Autodesk Inventor part; units mm, degrees
ref_plane "YZ Plane" through (0, 0, 0) normal (1, 0, 0) x (0, 1, 0)
ref_plane "XZ Plane" through (0, 0, 0) normal (0, 1, 0) x (-1, 0, 0)
ref_plane "XY Plane" through (0, 0, 0) normal (0, 0, 1) x (1, 0, 0)
sketch "Sketch1" plane through (0, 0, 0) normal (0, 1, 0) x (-1, 0, 0)
  line L0 (-0.2028, 19.4) -> (-0.2028, 32.1) construction
  line L1 (-2.584, 19.4) -> (-2.584, 32.1)
  line L2 (2.1785, 32.1) -> (2.1785, 19.4)
  arc A0 (-2.584, 19.4) -> (2.1785, 19.4) centre (-0.2028, 19.4) ccw
  arc A1 (2.1785, 32.1) -> (-2.584, 32.1) centre (-0.2028, 32.1) ccw
  line L3 (-0.2028, -19.4) -> (-0.2028, -32.1) construction
  line L4 (-2.584, -19.4) -> (-2.584, -32.1)
  line L5 (2.1785, -32.1) -> (2.1785, -19.4)
  arc A2 (2.1785, -19.4) -> (-2.584, -19.4) centre (-0.2028, -19.4) ccw
  arc A3 (-2.584, -32.1) -> (2.1785, -32.1) centre (-0.2028, -32.1) ccw
  line L6 (-51.0028, -76.2) -> (50.5972, -76.2)
  line L7 (50.5972, -76.2) -> (50.5972, 76.2)
  line L8 (50.5972, 76.2) -> (-51.0028, 76.2)
  line L9 (-51.0028, 76.2) -> (-51.0028, -76.2)
  line L10 (-51.0028, -76.2) -> (50.5972, 76.2) construction
  line L11 (50.5972, -76.2) -> (-51.0028, 76.2) construction
  line L12 (50.5972, 76.2) -> (50.5972, 50.8)
  line L13 (50.5972, 50.8) -> (25.1972, 50.8)
  line L14 (-51.0028, 76.2) -> (-51.0028, 50.8)
  line L15 (-51.0028, 50.8) -> (-25.6028, 50.8)
  line L16 (50.5972, -76.2) -> (50.5972, -50.8)
  line L17 (50.5972, -50.8) -> (25.1972, -50.8)
  line L18 (-51.0028, -76.2) -> (-51.0028, -50.8)
  line L19 (-51.0028, -50.8) -> (-25.6028, -50.8)
  circle A4 centre (25.1972, 50.8) radius 2.3813
  circle A5 centre (25.1972, -50.8) radius 2.3812
  circle A6 centre (-25.6028, 50.8) radius 2.3812
  circle A7 centre (-25.6028, -50.8) radius 2.3812
  arc A8 (-2.584, 31.6606) -> (-2.584, -31.6606) centre (-0.2028, 0) ccw
  arc A9 (2.1785, -31.6606) -> (2.1785, 31.6606) centre (-0.2028, 0) ccw
  point P0 (0, 0)
  dimension "d7" = 101.6
  dimension "d8" = 152.4
  dimension "d9" = 25.4
  dimension "d10" = 25.4
  dimension "d11" = 25.4
  dimension "d12" = 25.4
  dimension "d13" = 25.4
  dimension "d14" = 25.4
  dimension "d15" = 25.4
  dimension "d16" = 25.4
  dimension "d17" = 4.7625
  dimension "d18" = 4.7625
  dimension "d19" = 4.7625
  dimension "d20" = 4.7625
extrude "Extrusion1" add sketch "Sketch1" along normal blind 6.35 contours A0 L2 A9 L5 A2 L4 A8 L1 | L9 L8 L7 L6
sketch "Sketch2" plane through (0, 6.35, 0) normal (0, 1, 0) x (1, 0, 0)
  circle A0 centre (0, 0) radius 9.75
  dimension "d23" = 19.5
extrude "Extrusion2" cut sketch "Sketch2" against normal blind 6.35
sketch "Sketch3" plane through (0, 6.35, 0) normal (0, 1, 0) x (1, 0, 0)
  line L0 (-6.6401, -37.7246) -> (10.2278, -37.7246)
  line L1 (10.2278, -37.7246) -> (10.2278, -15.7747)
  line L2 (10.2278, -15.7747) -> (-6.6401, -15.7747)
  line L3 (-6.6401, -15.7747) -> (-6.6401, -37.7246)
  line L4 (-9.2351, 15.4742) -> (5.254, 15.4742)
  line L5 (5.254, 15.4742) -> (5.254, 41.8573)
  line L6 (5.254, 41.8573) -> (-9.2351, 41.8573)
  line L7 (-9.2351, 41.8573) -> (-9.2351, 15.4742)
  point P0 (0, 0)
extrude "Extrusion3" add sketch "Sketch3" against normal blind 6.35
sketch "Sketch4" plane through (0, 6.35, 0) normal (0, 1, 0) x (1, 0, 0)
  circle A0 centre (0, 0) radius 31.75
  line L0 (0, -31.75) -> (0, -25.75)
  line L1 (0, 31.75) -> (0, 25.75)
  circle A1 centre (0, -25.75) radius 2.3812
  circle A2 centre (0, 25.75) radius 2.3813
  line L2 (0, -22.75) -> (0, -28.75) construction
  line L3 (2.3812, -22.75) -> (2.3812, -28.75)
  line L4 (-2.3812, -28.75) -> (-2.3812, -22.75)
  arc A3 (2.3812, -22.75) -> (-2.3812, -22.75) centre (0, -22.75) ccw
  arc A4 (-2.3812, -28.75) -> (2.3812, -28.75) centre (0, -28.75) ccw
  line L5 (0, 22.75) -> (0, 28.75) construction
  line L6 (2.3813, 22.75) -> (2.3813, 28.75)
  line L7 (-2.3813, 28.75) -> (-2.3813, 22.75)
  arc A5 (-2.3813, 22.75) -> (2.3813, 22.75) centre (0, 22.75) ccw
  arc A6 (2.3813, 28.75) -> (-2.3813, 28.75) centre (0, 28.75) ccw
  dimension "d28" = 63.5
  dimension "d29" = 6
  dimension "d30" = 6
  dimension "d31" = 4.7625
  dimension "d32" = 4.7625
extrude "Extrusion4" cut sketch "Sketch4" against normal blind 6.35 contours A6 L6 A2 L1 | L1 A2 L7 A6 | A4 L4 A1 L0 | L0 A1 L3 A4 | A2 | A1 | L6 A5 L7 A2 | L4 A3 L3 A1
chamfer "Chamfer1" distance 25.4 angle 45 4 edges at (-50.5972, 3.175, 76.2) (51.0028, 3.175, 76.2) (-50.5972, 3.175, -76.2) (51.0028, 3.175, -76.2)
sketch "Sketch5" plane through (0, 6.35, 0) normal (0, 1, 0) x (1, 0, 0)
  line L0 (-50.5972, 50.8) -> (-50.5972, -50.8)
  circle A0 centre (-50.5972, 0) radius 28.575
  line L1 (51.0028, -50.8) -> (51.0028, 50.8)
  circle A1 centre (51.0028, 0) radius 28.575
  point P0 (0, 0)
  dimension "d38" = 57.15
  dimension "d39" = 57.15
extrude "Extrusion5" cut sketch "Sketch5" against normal blind 6.35
properties part number "motor mount plate"
Geometry check sheet. Reference: the model listing, model coordinates, mm. A direction names the side the tool comes from. Round coordinates to 2 decimals unless told otherwise and drop trailing zeros. Order: outer loops, then holes, each group sorted by start corner. A loop starts at its lowest first (then second) coordinate and runs counter-clockwise, first axis right, second up. Notation, with made-up numbers: M -23.75,54 L 16.25,54 A36 cw 16.25,88 Z; hole C 27,0.5 d10. An arc over 180 degrees is marked long. Answer in a Markdown table with one row per item. Add a question column.
Item 1: Sectioned sample at A-A, the plane x = 0. Enter the section's corners in (y, z).
Item 2: Material ranges on L1, parallel to Z at x = 0, y = 2; L2, parallel to X at y = 3.25, z = 0; L3, parallel to Z at x = 5, y = 3.75, recorded low to high. Write a range as [from, to].
Item 3: Sectioned sample at B-B, the plane z = 0. Enter the section's corners in (x, y).
Item 4: Sectioned sample at C-C, the plane y = 2.75. State how many separate pieces and enclosed holes the cut face has, plus the area to 3 significant figures.
Item 5: Depth check by flat-ended pin: pin 1 Ø22.5 at (x, z) = (0, 0) entering from +Y; pin 2 Ø3 at (y, z) = (3.5, -55) entering from -X; pin 3 Ø3 at (x, z) = (-25.2, 50.8) entering from -Y; pin 4 Ø1.8 at (y, z) = (4.5, -25) entering from +X. Enter the tip coordinate at first touch or a pass-through.
Item 6: Set-up check for faces 1 (the face through (-10, 6.35, 1)), 2 (the face through (0.05, 3.22, 20.37)): record each of +Z, -Z, +X, -X, +Y, -Y from which the full face is reachable in a straight line by a thin tool's end or side.
Filled in:
| question | item | result |
|---|---|---|
| 1 | outline | M 0,-76.2 L 6.35,-76.2 L 6.35,-31.13 L 0,-31.13 Z; M 0,-20.37 L 6.35,-20.37 L 6.35,-9.75 L 0,-9.75 Z; M 0,9.75 L 6.35,9.75 L 6.35,20.37 L 0,20.37 Z; M 0,31.13 L 6.35,31.13 L 6.35,76.2 L 0,76.2 Z |
| 2 | L1 | z = [-76.2, -31.13], [-20.37, -9.75], [9.75, 20.37], [31.13, 76.2] |
| 2 | L2 | x = [-22.02, -9.75], [9.75, 22.43] |
| 2 | L3 | z = [-76.2, -8.37], [8.37, 76.2] |
| 3 | outline | M -22.02,0 L -9.75,0 L -9.75,6.35 L -22.02,6.35 Z; M 9.75,0 L 22.43,0 L 22.43,6.35 L 9.75,6.35 Z |
| 4 | separate pieces | 1 |
| 4 | enclosed holes | 7 |
| 4 | area | 11,200 mm² |
| 5 | pin 1 | stops at y = 6.35 |
| 5 | pin 2 | stops at x = -47.9 |
| 5 | pin 3 | passes through |
| 5 | pin 4 | stops at x = 38.93 |
| 6 | face 1 | +Z, -Z, +X, -X, +Y |
| 6 | face 2 | +Y, -Y |
